Geometry check sheet. Reference: drawing and pictorial views, mm from the part's lowest x, y, z. Give positions to 0.01 mm unless a question says otherwise; leave off trailing zeros. Order: outer loops, then holes, each group sorted by start corner. A loop starts at its lowest first (then second) coordinate and runs counter-clockwise, first axis right, second up. Notation, with made-up numbers: (0.5, -22) - (59.5, -22) arc R23 cw to (59.5, 14) - close; hole circle Ø10 at (81.25, 58). An arc over 180 degrees is marked (long way). Answer as a JSON object with one key per item and string values.
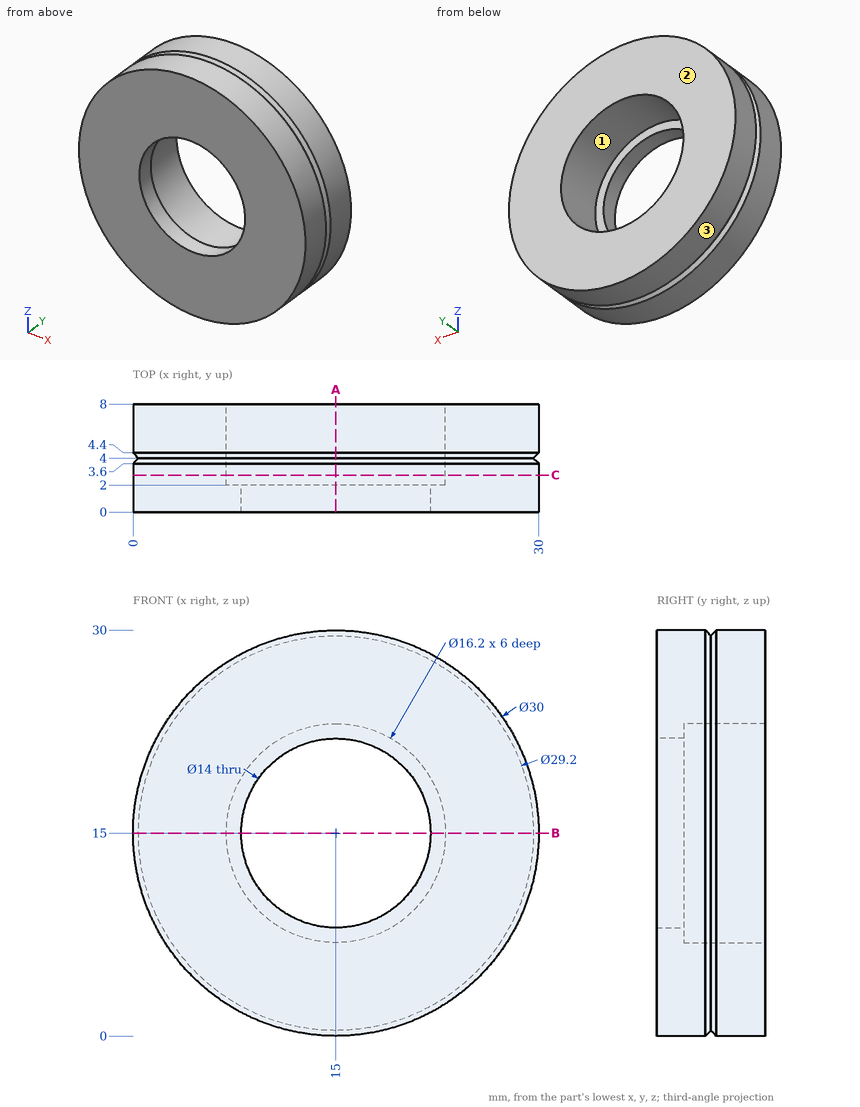
(1) Material ranges on line 1 along X through (y, z) = (1, 15); line 2 along X through (y, z) = (5.55, 15); line 3 along Z through (x, y) = (14, 5.25), recorded low to high. Write a range as [from, to].
Computed values:
{"line 1": "x = [0, 8], [22, 30]", "line 2": "x = [0, 6.9], [23.1, 30]", "line 3": "z = [0.03, 6.96], [23.04, 29.97]"}
(2) Release check for a two-part mould opening along Z. For the marked faces 1, 2 and 3 record: pulls with the +Z half, pulls with the -Z half, needs draft (parallel to the pull), parting line crosses it, or undercut.
Computed values:
{"face 1": "undercut", "face 2": "needs draft", "face 3": "parting line crosses it"}
(3) Section check A-A (x = 15). Record the cut outline in (y, z).
Computed values:
{"outline": "(0, 0) - (3.6, 0) - (4, 0.4) - (4.4, 0) - (8, 0) - (8, 6.9) - (2, 6.9) - (2, 8) - (0, 8) - close; (0, 22) - (2, 22) - (2, 23.1) - (8, 23.1) - (8, 30) - (4.4, 30) - (4, 29.6) - (3.6, 30) - (0, 30) - close"}
(4) Gauge pin test, flat ends, axial feed: pin 1 Ø14.5 at (x, z) = (15, 15) entering from +Y; pin 2 Ø4 at (y, z) = (2, 21.5) entering from +X; pin 3 Ø1.5 at (x, z) = (20, 15) entering from -Y; pin 4 Ø1 at (x, y) = (13, 4) entering from +Z. Record the tip position at first contact, or that the pin passes through.
Computed values:
{"pin 1": "stops at y = 2", "pin 2": "stops at x = 29.31", "pin 3": "passes through", "pin 4": "stops at z = 29.9"}
(5) Section check B-B (z = 15). Record the cut outline in (x, y).
Computed values:
{"outline": "(0, 0) - (8, 0) - (8, 2) - (6.9, 2) - (6.9, 8) - (0, 8) - (0, 4.4) - (0.4, 4) - (0, 3.6) - close; (22, 0) - (30, 0) - (30, 3.6) - (29.6, 4) - (30, 4.4) - (30, 8) - (23.1, 8) - (23.1, 2) - (22, 2) - close"}
(6) Section check C-C (y = 2.75). Record the cut outline in (x, z).
Computed values:
{"outline": "circle Ø30 at (15, 15); hole circle Ø16.2 at (15, 15)"}
